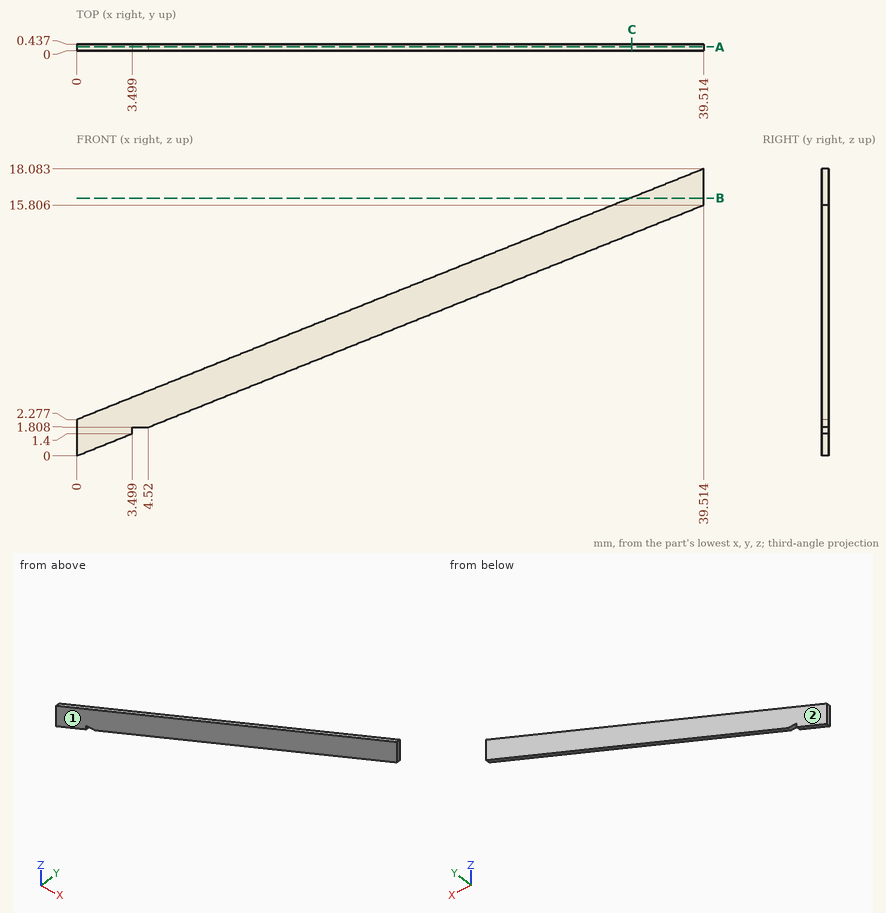
For this review, use the dimensioned drawing (mm, ordinates from the lowest corner) and the shaded views. Round coordinates to 2 decimals unless told otherwise and drop trailing zeros. Write each loop counter-clockwise with the first axis right and the second up, starting at its lowest first coordinate (ties: lowest second). Pieces come first, ordered by that corner, then holes. Notation, with made-up numbers: (39.25, 56) - (69.25, 56) arc R28 ccw to (69.25, 78) - close; hole circle Ø6 at (77.5, 77.5). An arc over 180 degrees is marked (long way). Use a Markdown table: item, result.
Q1. We need section C-C (x = 35). Give the boundary of the cut face in (y, z).
Derived:
| item | result |
|---|---|
| outline | (0, 14) - (0.44, 14) - (0.44, 16.28) - (0, 16.28) - close |
Q2. We need section B-B (z = 16.25). Give the boundary of the cut face in (x, y) (1 decimal).
Derived:
| item | result |
|---|---|
| outline | (34.9, 0) - (39.5, 0) - (39.5, 0.4) - (34.9, 0.4) - close |
Q3. Wall thickness on line 1 along X through (y, z) = (0.15, 1.5); line 2 along Z through (x, y) = (14, 0.1); line 3 along Z through (x, y) = (31.5, 0.1): over which ranges is each line inside the solid? List them lowest first.
Derived:
| item | result |
|---|---|
| line 1 | x = 0 to 3.5 |
| line 2 | z = 5.6 to 7.88 |
| line 3 | z = 12.6 to 14.88 |
Q4. We need section A-A (y = 0.25). Give the boundary of the cut face in (x, z) (1 decimal).
Derived:
| item | result |
|---|---|
| outline | (0, 0) - (3.5, 1.4) - (3.5, 1.8) - (4.5, 1.8) - (39.5, 15.8) - (39.5, 18.1) - (0, 2.3) - close |
Q5. Clearance check with a flat-ended pin moving along its axis: pin 1 (3 mm diameter, centred on x = 31, z = 11, fed in from -Y). State where the tip first meets the part, or that it passes through.
Derived:
| item | result |
|---|---|
| pin 1 | stops at y = 0 |
Q6. The part is to be moulded in two halves that separate along Y. For the marked faces 1 and 2, say which applies: pulls with the +Y half, pulls with the -Y half, needs draft (parallel to the pull), parting line crosses it, or undercut.
Derived:
| item | result |
|---|---|
| face 1 | pulls with the -Y half |
| face 2 | pulls with the +Y half |
